Work out the finished part from the listing and answer in its coordinate system (mm). Face numbers are marked on the shaded views. A direction names the side the tool comes from. Give positions to 0.01 mm unless a question says otherwise; leave off trailing zeros. Order: outer loops, then holes, each group sorted by start corner. A loop starts at its lowest first (then second) coordinate and runs counter-clockwise, first axis right, second up.
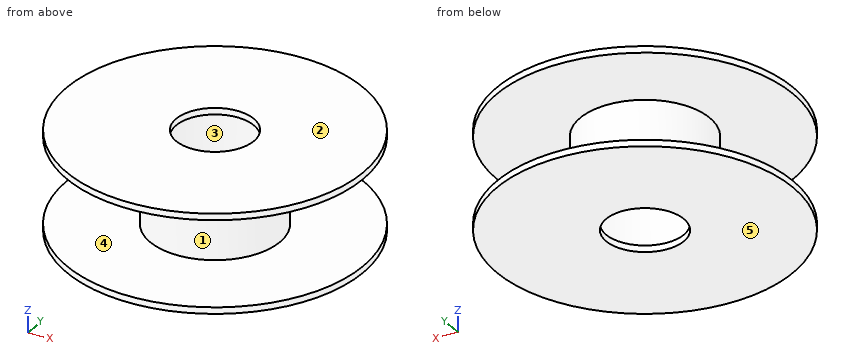
```python
from build123d import *

# Parameters (mm, degrees)
F0_R     = 101.6
F0_R_2   = 26.67
F1_DEPTH = 4.4196
F2_R     = 44.45
F2_R_2   = 26.67
F3_DEPTH = 58.9026
F5_DEPTH = 58.9026
F6_R     = 101.6
F6_R_2   = 44.45
F6_R_3   = 41.275
F6_R_4   = 26.67
F7_DEPTH = 4.4196


with BuildPart() as f1:
    # F0 (on Top) → F1 (new body)
    with BuildSketch(Plane.XY):
        Circle(F0_R)
        Circle(F0_R_2, mode=Mode.SUBTRACT)
    extrude(amount=F1_DEPTH)

    # F2 (on face) → F3 (join)
    with BuildSketch(Plane.XY.offset(4.4196)):
        Circle(F2_R)
        Circle(F2_R_2, mode=Mode.SUBTRACT)
    extrude(amount=F3_DEPTH)

    # F4 (on face) → F5 (cut, through all)
    with BuildSketch(Plane.XY.offset(63.3222)):
        with BuildLine():
            ThreePointArc((-41.275, 0), (0, -41.275), (41.275, 0))
            ThreePointArc((41.275, 0), (0, 41.275), (-41.275, 0))
        make_face()
    extrude(amount=-F5_DEPTH, mode=Mode.SUBTRACT)

    # F6 (on face) → F7 (join)
    with BuildSketch(Plane.XY.offset(63.3222)):
        Circle(F6_R)
        Circle(F6_R_2, mode=Mode.SUBTRACT)
        Circle(F6_R_2)
        Circle(F6_R_3, mode=Mode.SUBTRACT)
        Circle(F6_R_3)
        Circle(F6_R_4, mode=Mode.SUBTRACT)
    extrude(amount=F7_DEPTH)


solid = f1.part
```
1. The part is cut by section C-C (y = 37). Write down the section's boundary in (x, z).
Findings below:
outline: (-94.62, 0) - (94.62, 0) - (94.62, 4.42) - (24.63, 4.42) - (24.63, 63.32) - (94.62, 63.32) - (94.62, 67.74) - (-94.62, 67.74) - (-94.62, 63.32) - (-24.63, 63.32) - (-24.63, 4.42) - (-94.62, 4.42) - close; hole (-18.29, 4.42) - (18.29, 4.42) - (18.29, 63.32) - (-18.29, 63.32) - close
2. The part is cut by section A-A (x = 0). Write down the section's boundary in (y, z) (3 decimals), then the cut area to 3 significant figures.
Findings below:
outline: (-101.6, 0) - (-26.67, 0) - (-26.67, 4.42) - (-41.275, 4.42) - (-41.275, 63.322) - (-26.67, 63.322) - (-26.67, 67.742) - (-101.6, 67.742) - (-101.6, 63.322) - (-44.45, 63.322) - (-44.45, 4.42) - (-101.6, 4.42) - close; (26.67, 0) - (101.6, 0) - (101.6, 4.42) - (44.45, 4.42) - (44.45, 63.322) - (101.6, 63.322) - (101.6, 67.742) - (26.67, 67.742) - (26.67, 63.322) - (41.275, 63.322) - (41.275, 4.42) - (26.67, 4.42) - close
area: 1,700 mm2
3. Straight lines are drawn through the part: probe 1 along Y at (x, z) = (0, 65); probe 2 along Z at (x, y) = (-62, 11.5); probe 3 along Y at (x, z) = (0, 21) (3 decimals). For each, find the intervals that lie inside material, in ascending order.
Findings below:
probe 1: y = -101.6 to -26.67, 26.67 to 101.6
probe 2: z = 0 to 4.42, 63.32 to 67.74
probe 3: y = -44.45 to -41.275, 41.275 to 44.45
4. Which of the six approach directions +Z, -Z, +X, -X, +Y, -Y give full straight-line access (tool end or side, diameter ignored) to the marked faces 4 and 5?
Findings below:
face 4: none
face 5: -Z, +X, -X, +Y, -Y
5. The mould has two halves that part along Y. Classify the marked faces 1, 2 and 3: pulls with the +Y half, pulls with the -Y half, needs draft (parallel to the pull), parting line crosses it, or undercut.
Findings below:
face 1: parting line crosses it
face 2: needs draft
face 3: undercut
6. The part is cut by section D-D (z = 11). Write down the section's boundary in (x, y) (3 decimals).
Findings below:
outline: circle Ø88.9 at (0, 0); hole circle Ø82.55 at (0, 0)
7. Given P1, Ø5, axis at x = -4, z = 34, coming from the -Y side; P2, Ø12, axis at y = 29.5, z = 14, coming from the -X side; P3, Ø1.5, axis at y = 24, z = 58, coming from the +X side, each flat-ended and moving along its own axis, determine where each tip first touches the part or whether it passes through.
Findings below:
P1: stops at y = -44.42
P2: stops at x = -37.73
P3: stops at x = 37.88
